Can you work these out from the model? Positions are in its coordinate system, mm. Face numbers are marked on the shaded views. A direction names the side the tool comes from. Coordinates: 2 decimals unless noted, no trailing zeros. Order: outer loops, then holes, each group sorted by start corner. A loop starts at its lowest first (then second) coordinate and runs counter-clockwise, first axis right, second up. Notation, with made-up numbers: (8.25, 39.25) -> (15.25, 39.25) arc R17 cw to (15.25, 50.25) -> close; hole circle Ø4 at (-5.75, 63). An arc over 180 degrees is marked (long way). Write item = value, one per line.
```python
from build123d import *

# Parameters (mm, degrees)
SKETCH1_W               = 40.4
SKETCH1_H               = 42.6
BOSS_EXTRUDE1_DEPTH     = 1.6
SKETCH2_R               = 1.5
CUT_EXTRUDE1_DEPTH      = 30.3988095
CUT_EXTRUDE_THIN2_DEPTH = 0.1
FILLET1_R               = 3
SKETCH3_W               = 4
SKETCH3_H               = 5.25
BOSS_EXTRUDE2_DEPTH     = 2.7
SKETCH4_W               = 6
SKETCH4_H               = 6
BOSS_EXTRUDE3_DEPTH     = 1
SKETCH6_R               = 0.5
CUT_EXTRUDE2_DEPTH      = 30.479145171


with BuildPart() as part:
    # Sketch1 → Boss-Extrude1 (new body)
    with BuildSketch(Plane(origin=(0, 0, 0), x_dir=(1, 0, 0), z_dir=(0, 1, 0))):
        Rectangle(SKETCH1_W, SKETCH1_H)
    extrude(amount=BOSS_EXTRUDE1_DEPTH)

    # Sketch2 → Cut-Extrude1 (cut, through all)
    with BuildSketch(Plane(origin=(0, 1.6, 0), x_dir=(1, 0, 0), z_dir=(0, 1, 0))):
        with Locations(Location((12.867890888, 13.568617619, 0), (0, 0, 270))):
            Circle(SKETCH2_R)
        with Locations(Location((-12.867890888, -13.568617619, 0), (0, 0, 270))):
            Circle(SKETCH2_R)
    extrude(amount=-CUT_EXTRUDE1_DEPTH, mode=Mode.SUBTRACT)

    # Sketch5 → Cut-Extrude-Thin2 (cut)
    with BuildSketch(Plane(origin=(0, 1.6, 0), x_dir=(1, 0, 0), z_dir=(0, 1, 0))):
        Polygon((-15.321320344, 20.3), (-19.2, 16.421320344), (-19.2, -16.421320344), (-15.321320344, -20.3), (15.321320344, -20.3), (19.2, -16.421320344), (19.2, 16.421320344), (15.321320344, 20.3), align=None)
        Polygon((-14.078679656, 17.3), (-16.2, 15.178679656), (-16.2, -15.178679656), (-14.078679656, -17.3), (14.078679656, -17.3), (16.2, -15.178679656), (16.2, 15.178679656), (14.078679656, 17.3), align=None, mode=Mode.SUBTRACT)
    extrude(amount=-CUT_EXTRUDE_THIN2_DEPTH, mode=Mode.SUBTRACT)

    # Fillet1
    fillet1_edges = [part.edges().sort_by_distance(p)[0] for p in [
        (-20.2, 0.8, -21.3),
        (20.2, 0.8, -21.3),
        (20.2, 0.8, 21.3),
        (-20.2, 0.8, 21.3),
    ]]
    fillet(fillet1_edges, radius=FILLET1_R)

    # Sketch3 → Boss-Extrude2 (add)
    with BuildSketch(Plane(origin=(0, 1.6, 0), x_dir=(1, 0, 0), z_dir=(0, 1, 0))):
        with Locations((-9.2, 9.925)):
            Rectangle(SKETCH3_W, SKETCH3_H)
    extrude(amount=BOSS_EXTRUDE2_DEPTH)

    # Sketch4 → Boss-Extrude3 (add)
    with BuildSketch(Plane(origin=(0, 1.6, 0), x_dir=(1, 0, 0), z_dir=(0, 1, 0))):
        with Locations((0, -6)):
            Rectangle(SKETCH4_W, SKETCH4_H)
    extrude(amount=BOSS_EXTRUDE3_DEPTH)

    # Sketch6 → Cut-Extrude2 (cut, through all)
    with BuildSketch(Plane(origin=(0, 1.6, 0), x_dir=(1, 0, 0), z_dir=(0, 1, 0))):
        with Locations(Location((-3.75, 14.3, 0), (0, 0, 270))):
            Circle(SKETCH6_R)
        with Locations(Location((-1.25, 14.3, 0), (0, 0, 270))):
            Circle(SKETCH6_R)
        with Locations(Location((1.25, 14.3, 0), (0, 0, 270))):
            Circle(SKETCH6_R)
        with Locations(Location((3.75, 14.3, 0), (0, 0, 270))):
            Circle(SKETCH6_R)
    extrude(amount=-CUT_EXTRUDE2_DEPTH, mode=Mode.SUBTRACT)


solid = part.part
```
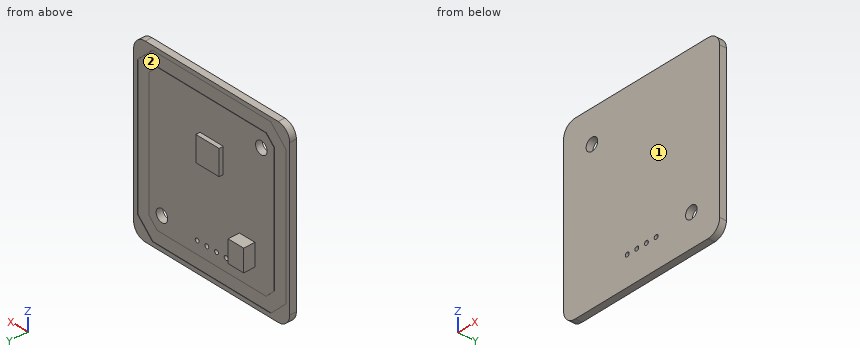
Item 1: I want a section at B-B, the plane x = 3.75. Please give me the cut outline in (y, z), plus the area to 3 significant figures.
A:
outline = (0, -21.3) -> (1.6, -21.3) -> (1.6, -20.3) -> (1.5, -20.3) -> (1.5, -17.3) -> (1.6, -17.3) -> (1.6, -14.8) -> (0, -14.8) -> close; (0, -13.8) -> (1.6, -13.8) -> (1.6, 17.3) -> (1.5, 17.3) -> (1.5, 20.3) -> (1.6, 20.3) -> (1.6, 21.3) -> (0, 21.3) -> close
area = 66.0 mm2
Item 2: I want a section at D-D, the plane x = 9. Please give me the cut outline in (y, z).
A:
outline = (0, -21.3) -> (1.6, -21.3) -> (1.6, -20.3) -> (1.5, -20.3) -> (1.5, -17.3) -> (1.6, -17.3) -> (1.6, 17.3) -> (1.5, 17.3) -> (1.5, 20.3) -> (1.6, 20.3) -> (1.6, 21.3) -> (0, 21.3) -> close
Item 3: I'm going to push flat-ended pins straight in: P1, Ø9.5, axis at x = 6, z = -1, coming from the +Y side; P2, Ø1.4, axis at x = -9.5, y = 3, coming from the -Z side; P3, Ø2, axis at y = 3.5, z = -8.5, coming from the +X side; P4, Ø2, axis at y = 3, z = 0, coming from the -X side. Where does each tip first touch, or does it pass through?
A:
P1 = 1.6
P2 = -12.55
P3 = -7.2
P4 = through
Item 4: If I drill on probe 1 along X at (y, z) = (0.75, -14.3); probe 2 along Z at (x, y) = (-14, 1.4); probe 3 along X at (y, z) = (0.7, -13.5), over which ranges is the centre line in solid material (lowest first)?
A:
probe_1 = -20.2 to -4.25, -3.25 to -1.75, -0.75 to 0.75, 1.75 to 3.25, 4.25 to 11.56, 14.18 to 20.2
probe_2 = -21.3 to 12.58, 14.55 to 21.3
probe_3 = -20.2 to 11.37, 14.37 to 20.2
Item 5: I want a section at C-C, the plane z = 14.5. Please give me the cut outline in (x, y), plus the area to 3 significant figures.
A:
outline = (-20.2, 0) -> (-14.04, 0) -> (-14.04, 1.6) -> (-16.2, 1.6) -> (-16.2, 1.5) -> (-19.2, 1.5) -> (-19.2, 1.6) -> (-20.2, 1.6) -> close; (-11.69, 0) -> (20.2, 0) -> (20.2, 1.6) -> (19.2, 1.6) -> (19.2, 1.5) -> (16.2, 1.5) -> (16.2, 1.6) -> (-11.69, 1.6) -> close
area = 60.3 mm2
Item 6: For the marked faces 1 and 2, which set-ups out of +Z, -Z, +X, -X, +Y, -Y let a thin tool reach every point of the face, with its end or its side?
A:
face_1 = +Z, -Z, +X, -X, -Y
face_2 = +Y
Item 7: I want a section at A-A, the plane y = 2.1. Please give me the cut outline in (x, z), plus the area to 3 significant figures.
A:
outline = (-11.2, -12.55) -> (-7.2, -12.55) -> (-7.2, -7.3) -> (-11.2, -7.3) -> close; (-3, 3) -> (3, 3) -> (3, 9) -> (-3, 9) -> close
area = 57.0 mm2
